Source: CAD feature listing. Evaluate the final solid. Frame: model axes, mm. Face numbers are marked on the shaded views. A direction names the side the tool comes from. Give positions to 0.01 mm unless a question says otherwise; leave off trailing zeros. Order: outer loops, then holes, each group sorted by start corner. A loop starts at its lowest first (then second) coordinate and runs counter-clockwise, first axis right, second up. Notation, with made-up numbers: M 35.5,13.5 L 54.5,13.5 A25 cw 54.5,35.5 Z; hole C 24.5,-35.5 d3. An arc over 180 degrees is marked long. Use CSV: the item, a comma, the result in double quotes. Start each with the question number.
Item 1: Section query A-A on x = 40. Return loops of the section in (y, z), and give its area (3 significant figures).
Item 2: Section query D-D on z = 12.5. Return loops of the section in (x, y), and give its area (4 significant figures).
Item 3: Access query for the marked faces 1, 2, 3 and 4. Directions: +Z, -Z, +X, -X, +Y, -Y. A direction counts if a zero-diameter tool reaches every point of the face in a straight line with its end or side. Return the directions, or none.
Item 4: Pull-direction query (X, two-part tool) for the marked faces 5, 6 and 7; classes: +X half, -X half, draft (parallel to the pull), parting line (faces both ways), or undercut.
Item 5: First-contact query: pin 1 (12 mm diameter, centred on x = 40, y = -35, fed in from -Z); pin 2 (22.5 mm diameter, centred on y = -39, z = 7, fed in from +X); pin 3 (3 mm diameter, centred on x = -8.5, z = 6, fed in from -Y); pin 4 (9 mm diameter, centred on x = -40, z = 24.61, fed in from +Y). Flat tips, straight axial feed; report the tip coordinate or a pass-through.
Item 6: Section query B-B on y = -35. Return loops of the section in (x, z).
Item 7: Ray query, probe 1 along Z at (x, y) = (40, -3); probe 2 along Z at (x, y) = (-40, -7); probe 3 along Y at (x, z) = (40, -22). Return the intervals inside material, ascending. Write a range as from..to.
Item 8: Section query C-C on x = 20. Return loops of the section in (y, z), and give its area (3 significant figures).
from build123d import *

# Parameters (mm, degrees)
F0_W     = 120
F0_H     = 15
F0_H_2   = 13.18299
F0_H_3   = 51.81701
F0_R     = 5
F1_DEPTH = 10
F2_W     = 120
F2_H     = 10
F3_DEPTH = 45
F4_R     = 5
F4_R_2   = 5.25369
F5_DEPTH = 25
F6_W     = 10
F6_H     = 55
F7_DEPTH = 45
F9_DEPTH = 10


with BuildPart() as f1:
    # F0 (on Front) → F1 (new body)
    with BuildSketch(Plane.XZ):
        with Locations((0, -32.5)):
            Rectangle(F0_W, F0_H)
        with Locations((0, -18.408505)):
            Rectangle(F0_W, F0_H_2)
        with Locations((0, 14.091495)):
            Rectangle(F0_W, F0_H_3)
        with Locations((-40, 24.60571)):
            Circle(F0_R, mode=Mode.SUBTRACT)
        with Locations((40, 24.445876)):
            Circle(F0_R, mode=Mode.SUBTRACT)
    extrude(amount=F1_DEPTH)

    # F2 (on face) → F3 (join)
    with BuildSketch(Plane.XZ.offset(10)):
        with Locations((0, -20)):
            Rectangle(F2_W, F2_H)
    extrude(amount=F3_DEPTH)

    # F4 (on face) → F5 (cut)
    with BuildSketch(Plane.XY.offset(-15)):
        with Locations((-40, -35)):
            Circle(F4_R)
        with Locations((40, -35)):
            Circle(F4_R_2)
    extrude(amount=-F5_DEPTH, mode=Mode.SUBTRACT)

    # F6 (on face) → F7 (join)
    with BuildSketch(Plane.XZ.offset(10)):
        with Locations((0, 12.5)):
            Rectangle(F6_W, F6_H)
    extrude(amount=F7_DEPTH)

    # F8 (on face) → F9 (cut)
    with BuildSketch(Plane.YZ.offset(5)):
        Polygon((-55, -15), (-10, 40), (-55, 40), align=None)
    extrude(amount=-F9_DEPTH, mode=Mode.SUBTRACT)


solid = f1.part
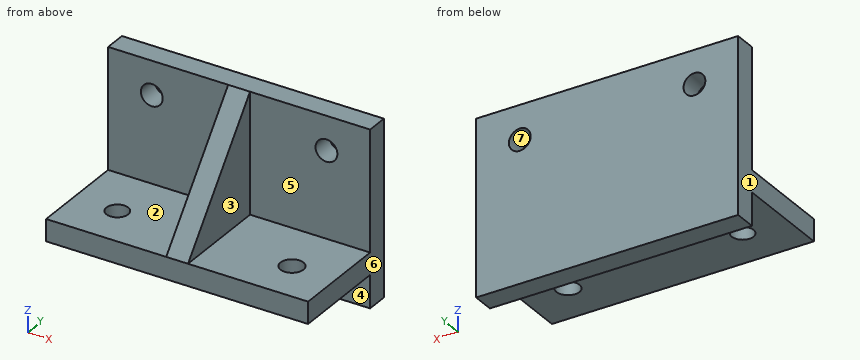
Verdict:
1,outline,"M -55,-25 L -40.25,-25 L -40.25,-15 L -55,-15 Z; M -29.75,-25 L -10,-25 L -10,-40 L 0,-40 L 0,19.45 L -10,19.45 L -10,-15 L -29.75,-15 Z; M -10,29.45 L 0,29.45 L 0,40 L -10,40 Z"
1,area,"1,040 mm2"
2,outline,"M -60,-10 L -5,-10 L -5,-32.5 L 5,-32.5 L 5,-10 L 60,-10 L 60,0 L -60,0 Z"
2,area,"1,425 mm2"
3,face 1,"+Z, -Z, -X, +Y, -Y"
3,face 2,"+Z, -X, -Y"
3,face 3,"+Z, +X, -Y"
3,face 4,"-Z, +X, -X, -Y"
4,face 5,"draft"
4,face 6,"+X half"
4,face 7,"undercut"
5,pin 1,"z = -25"
5,pin 2,"x = 5"
5,pin 3,"y = -10"
5,pin 4,"through"
6,outline,"M -60,-25 L -45,-25 L -45,-15 L -60,-15 Z; M -35,-25 L 34.75,-25 L 34.75,-15 L 5,-15 L 5,9.44 L -5,9.44 L -5,-15 L -35,-15 Z; M 45.25,-25 L 60,-25 L 60,-15 L 45.25,-15 Z"
7,probe 1,"-40..19.45, 29.45..40"
7,probe 2,"-40..19.61, 29.61..40"
7,probe 3,"-55..-40.25, -29.75..0"
8,outline,"M -55,-25 L -10,-25 L -10,-40 L 0,-40 L 0,40 L -10,40 L -10,-15 L -55,-15 Z"
8,area,"1,250 mm2"
